from build123d import *

# Parameters (mm, degrees)
F0_W     = 161.764927
F0_H     = 96.818306
F1_DEPTH = 84.328
F2_R     = 21.280915
F3_DEPTH = 84.329
F4_R     = 6.35
F5_DEPTH = 96.819306


with BuildPart() as f1:
    # F0 (on Top) → F1 (new body)
    with BuildSketch(Plane.XY):
        with Locations((17.771822, 6.286327)):
            Rectangle(F0_W, F0_H)
    extrude(amount=F1_DEPTH)

    # F2 (on face) → F3 (cut, through all)
    with BuildSketch(Plane.XY.offset(84.328)):
        with Locations((23.939807, 4.083021)):
            Circle(F2_R)
    extrude(amount=-F3_DEPTH, mode=Mode.SUBTRACT)

    # F4 (on face) → F5 (cut, through all)
    with BuildSketch(Plane.XZ.offset(42.122826)):
        with Locations((-37.710642, 51.287621)):
            Circle(F4_R)
    extrude(amount=-F5_DEPTH, mode=Mode.SUBTRACT)


solid = f1.part
Check sheet for the modelled part. Datum: model origin and axes. Units: mm. Give positions to 0.01 mm unless a question says otherwise; leave off trailing zeros. Loops run counter-clockwise (first coordinate to the right, second up) from the corner with the lowest first, then second, coordinate; pieces in that order, holes last. Notation, with made-up numbers: M -34,79.25 L -4,79.25 A32 ccw -4,106.25 Z; hole C 82.5,-40 d7. An arc over 180 degrees is marked long. Return JSON: item names as keys, results as strings. Group by question number.
1. Go/stop test with a flat-tipped pin: pin 1 (8 mm diameter, centred on x = -2, y = 12, fed in from -Z). Record where the tip stops, or that it passes through.
2. Thickness scan on L1, parallel to X at y = -3.5, z = 54; L2, parallel to Y at x = 21, z = 71.5; L3, parallel to Y at x = 43, z = 77. Record the ranges inside material, lowest first.
3. Mould release check, pull along Z, two halves, no side actions. Record for faces 1 (the cylindrical face through (-42.75, 5.609, 47.424)), 2 (the flat face through (-1, 7, 0)), 3 (the flat face through (-63.111, 6, 42)): released by +Z, released by -Z, zero draft, split by the parting line, or undercut.
4. Cross-section at C-C on z = 37. Record the boundary of the cut face in (x, y).
5. Cross-section at B-B on x = 21. Record the boundary of the cut face in (y, z).
6. Cross-section at D-D on y = 23.5. Record the boundary of the cut face in (x, z).
7. Cross-section at A-A on y = 6.5. Record the boundary of the cut face in (x, z).
Return value:
{
 "1": {"pin 1": "z = 0"},
 "2": {"L1": "-63.11 to -43.45, -31.97 to 4.06, 43.82 to 98.65", "L2": "-42.12 to -16.99, 25.16 to 54.7", "L3": "-42.12 to -5.38, 13.55 to 54.7"},
 "3": {"face 1": "undercut", "face 2": "released by -Z", "face 3": "zero draft"},
 "4": {"outline": "M -63.11,-42.12 L 98.65,-42.12 L 98.65,54.7 L -63.11,54.7 Z; hole C 23.94,4.08 d42.56"},
 "5": {"outline": "M -42.12,0 L -16.99,0 L -16.99,84.33 L -42.12,84.33 Z; M 25.16,0 L 54.7,0 L 54.7,84.33 L 25.16,84.33 Z"},
 "6": {"outline": "M -63.11,0 L 15.23,0 L 15.23,84.33 L -63.11,84.33 Z; M 32.65,0 L 98.65,0 L 98.65,84.33 L 32.65,84.33 Z; hole C -37.71,51.29 d12.7"},
 "7": {"outline": "M -63.11,0 L 2.8,0 L 2.8,84.33 L -63.11,84.33 Z; M 45.08,0 L 98.65,0 L 98.65,84.33 L 45.08,84.33 Z; hole C -37.71,51.29 d12.7"}
}
